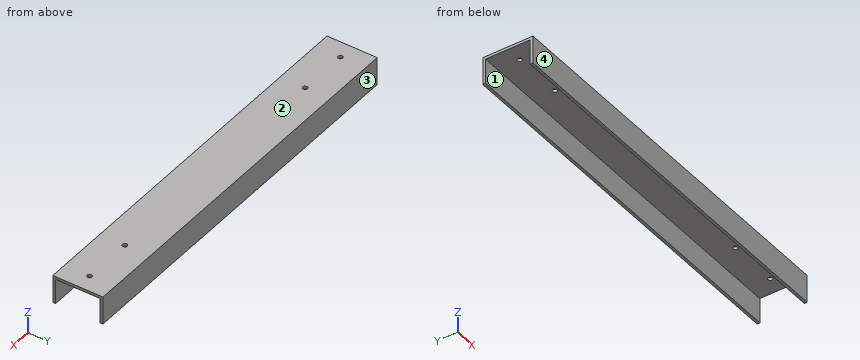
Autodesk Inventor part; units mm, degrees
ref_plane "YZ Plane" through (0, 0, 0) normal (1, 0, 0) x (0, 1, 0)
ref_plane "XZ Plane" through (0, 0, 0) normal (0, 1, 0) x (-1, 0, 0)
ref_plane "XY Plane" through (0, 0, 0) normal (0, 0, 1) x (1, 0, 0)
sketch "Sketch1" plane through (0, 0, 0) normal (0, 0, 1) x (1, 0, 0)
  line L0 (-350, 45) -> (350, 45)
  line L1 (-350, -45) -> (350, -45)
  line L2 (-350, 45) -> (-350, -45)
  line L3 (350, 45) -> (350, -45)
  line L4 (350, -45) -> (-350, 45) construction
  line L5 (-350, -45) -> (350, 45) construction
  point P0 (0, 0)
  point P1 (0, 0)
  dimension "d8" = 700
  dimension "d9" = 90
extrude "Extrusion1" add sketch "Sketch1" against normal blind 50
shell "Shell1" thickness 5 removed faces 3 at (350, 15, -16.6667) at (-350, -15, -16.6667) at (116.6667, 15, -50)
sketch "Sketch3" plane through (0, 0, 0) normal (0, 0, 1) x (1, 0, 0)
  point P0 (0, 0)
  point P1 (320, 0)
  point P2 (230, 0)
  dimension "d11" = 320
  dimension "d12" = 90
hole "Hole1" at (320, 0, 0) at (230, 0, 0) direction (0, 0, -1) diameter 8.376 end through all
pattern_circular "Circular Pattern1" count 2 over 360 about axis through (0, 0, -10) along (0, 0, 1) of "Hole1"
properties part number "ADSK-MH-10011" material "Steel, Mild"
CAD build for the part. Positions are in the model's coordinates, mm. Face numbers are marked on the shaded views. Coordinates: 2 decimals unless noted, no trailing zeros. Order: outer loops, then holes, each group sorted by start corner. A loop starts at its lowest first (then second) coordinate and runs counter-clockwise, first axis right, second up. Notation, with made-up numbers: M 11.5,-14.75 L 68.5,-14.75 A26 cw 68.5,7.25 Z; hole C -14,19.25 d4. An arc over 180 degrees is marked long. Answer as CSV lines item,"result".
1) Cut at B-B (x = 286.5). List the corners of the cut face in (y, z), then the cut area to 3 significant figures.
Verdict:
outline,"M -45,-50 L -40,-50 L -40,-5 L 40,-5 L 40,-50 L 45,-50 L 45,0 L -45,0 Z"
area,"900 mm2"
2) Drill centre lines: L1, parallel to X at y = 0, z = -1.65; L2, parallel to Y at x = 214, z = -21.5; L3, parallel to Z at x = 55.5, y = -24. Where is each one in solid material? Low to high. Write a range as from..to.
Verdict:
L1,"-350..-324.19, -315.81..-234.19, -225.81..225.81, 234.19..315.81, 324.19..350"
L2,"-45..-40, 40..45"
L3,"-5..0"
3) Flat gauge pins, fed straight in: P1, Ø5, axis at x = -320, y = 0, coming from the -Z side; P2, Ø12, axis at x = 260.5, y = 3.5, coming from the -Z side. Where does each tip first touch, or does it go through?
Verdict:
P1,"through"
P2,"z = -5"
4) Mould opens along Y. For the marked faces 1, 2, 3 and 4 say: released by +Y, released by -Y, zero draft, split by the parting line, or undercut.
Verdict:
face 1,"undercut"
face 2,"zero draft"
face 3,"released by +Y"
face 4,"released by -Y"
5) Cut at C-C (y = -33). List the corners of the cut face in (x, z), then the cut area to 3 significant figures.
Verdict:
outline,"M -350,-5 L 350,-5 L 350,0 L -350,0 Z"
area,"3,500 mm2"
6) Cut at A-A (z = -36.5). List the corners of the cut face in (x, y).
Verdict:
outline,"M -350,-45 L 350,-45 L 350,-40 L -350,-40 Z; M -350,40 L 350,40 L 350,45 L -350,45 Z"
